Verification items for this drawing (mm, ordinates from the low corner). A direction names the side the tool comes from. Round coordinates to 2 decimals unless told otherwise and drop trailing zeros. Order: outer loops, then holes, each group sorted by start corner. A loop starts at its lowest first (then second) coordinate and runs counter-clockwise, first axis right, second up. Notation, with made-up numbers: (-23, -28.75) - (11, -28.75) arc R6 ccw to (11, -17.75) - close; hole circle Ø11 at (17.5, -20.75). An arc over 180 degrees is marked (long way). Use a Markdown table: item, result. Add a question column.
(1) Section check B-B on x = 120.5. Record the boundary of the cut face in (y, z).
(2) Section check C-C on z = 50. Record the boundary of the cut face in (x, y).
(3) Section check D-D on y = 43. Record the boundary of the cut face in (x, z).
(4) Mould release check, pull along Z, two halves, no side actions. Record for the marked faces 4, 5, 6 and 7: released by +Z, released by -Z, zero draft, split by the parting line, or undercut.
(5) Thickness scan on line 1 along Z through (x, y) = (186.5, 168); line 2 along Y through (x, z) = (62, 50); line 3 along Y through (x, z) = (142, 33.5) (1 decimal). Record the ranges inside material, lowest first. Write a range as [from, to].
(6) Section check A-A on x = 170. Record the boundary of the cut face in (y, z).
(7) Gauge pin test, flat ends, axial feed: P1, Ø8, axis at x = 214.5, z = 47.5, coming from the +Y side; P2, Ø8, axis at x = 219, y = 111.5, coming from the -Z side; P3, Ø12, axis at x = 178, z = 81, coming from the +Y side; P4, Ø16, axis at x = 328.5, z = 81, coming from the -Y side. Record the tip position at first contact, or that the pin passes through.
(8) Access from +Z, -Z, +X, -X, +Y, -Y to the whole of each face (thin tool, end or side, straight path). Record for the marked faces 1, 2 and 3.
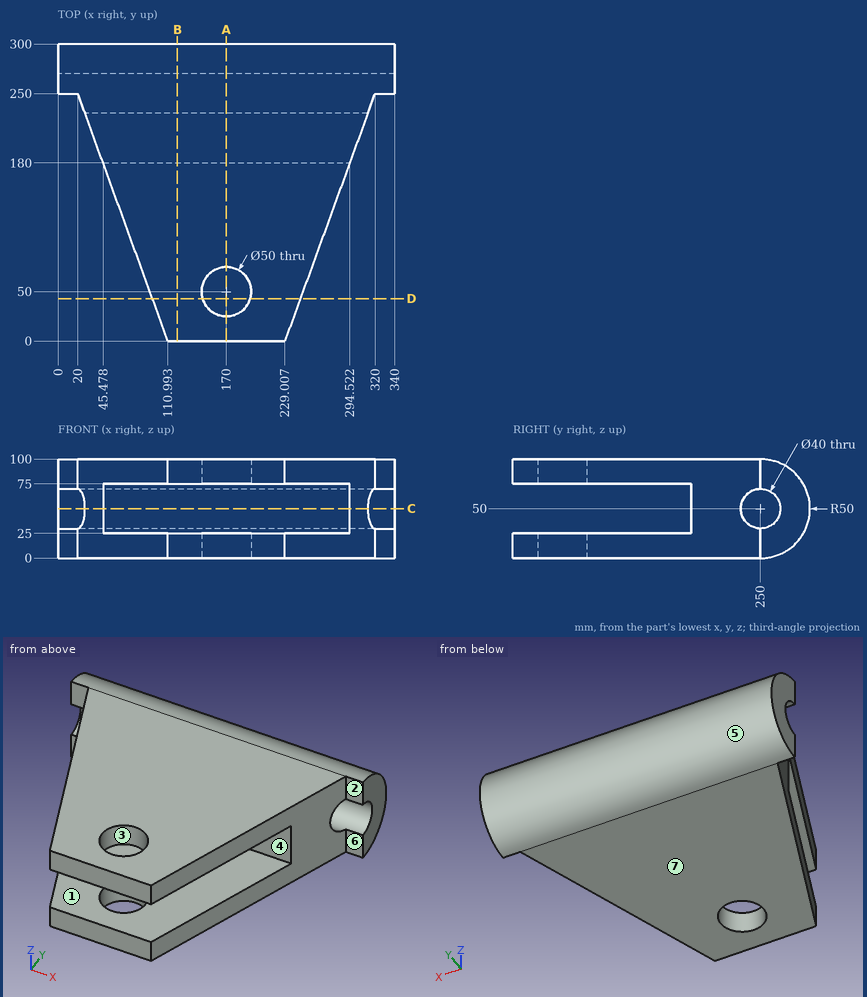
Check sheet entries:
| question | item | result |
|---|---|---|
| 1 | outline | (0, 0) - (250, 0) arc R50 ccw to (250, 100) - (0, 100) - (0, 75) - (180, 75) - (180, 25) - (0, 25) - close; hole circle Ø40 at (250, 50) |
| 2 | outline | (0, 270) - (340, 270) - (340, 300) - (0, 300) - close; (27.28, 230) - (45.48, 180) - (294.52, 180) - (312.72, 230) - close |
| 3 | outline | (95.34, 0) - (146, 0) - (146, 25) - (95.34, 25) - close; (95.34, 75) - (146, 75) - (146, 100) - (95.34, 100) - close; (194, 0) - (244.66, 0) - (244.66, 25) - (194, 25) - close; (194, 75) - (244.66, 75) - (244.66, 100) - (194, 100) - close |
| 4 | face 4 | undercut |
| 4 | face 5 | split by the parting line |
| 4 | face 6 | zero draft |
| 4 | face 7 | released by -Z |
| 5 | line 1 | z = [0, 25], [75, 100] |
| 5 | line 2 | y = [180, 230], [270, 300] |
| 5 | line 3 | y = [180, 238.7], [261.3, 297.2] |
| 6 | outline | (0, 0) - (25, 0) - (25, 25) - (0, 25) - close; (0, 75) - (25, 75) - (25, 100) - (0, 100) - close; (75, 0) - (250, 0) arc R50 ccw to (250, 100) - (75, 100) - (75, 75) - (180, 75) - (180, 25) - (75, 25) - close; hole circle Ø40 at (250, 50) |
| 7 | P1 | stops at y = 300 |
| 7 | P2 | stops at z = 0 |
| 7 | P3 | stops at y = 293.3 |
| 7 | P4 | stops at y = 250 |
| 8 | face 1 | +X, -X, -Y |
| 8 | face 2 | +Z, -Z, +X, -Y |
| 8 | face 3 | +Z, -Z |
